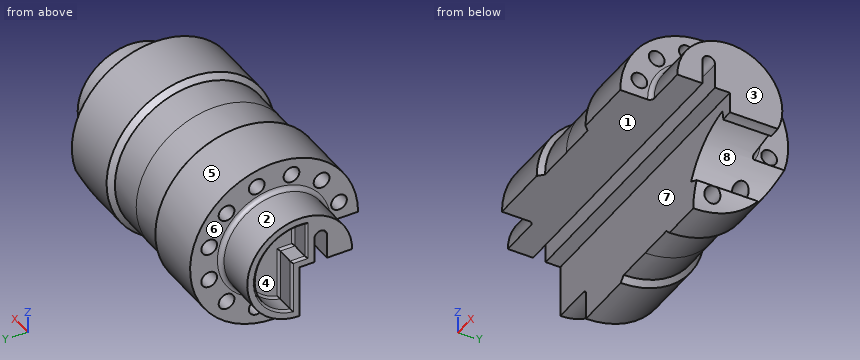
```python
from build123d import *

# Parameters (mm, degrees)
SKETCH2_W               = 86.249778207
SKETCH2_H               = 59.255694893
CUT_EXTRUDE1_DEPTH      = 1
CUT_EXTRUDE1_DEPTH_BACK = 139
CUT_EXTRUDE2_REACH      = 42
SKETCH4_R               = 3.75
CUT_EXTRUDE3_DEPTH      = 139
CUT_EXTRUDE4_DEPTH      = 10
FILLET1_R               = 1


with BuildPart() as part:
    # Sketch1 → Revolve1 (revolve)
    with BuildSketch(Plane(origin=(0, 0, 0), x_dir=(1, 0, 0), z_dir=(0, 1, 0))):
        with BuildLine():
            Line((-71.076656526, -28.85165756), (-71.076656526, -3.85165756))
            Line((-71.076656526, -3.85165756), (-52.076656526, -3.85165756))
            ThreePointArc((-52.076656526, -3.85165756), (-50.662442964, -3.265871122), (-50.076656526, -1.85165756))
            Line((-50.076656526, -1.85165756), (-50.076656526, 11.14834244))
            Line((-50.076656526, 11.14834244), (-21.576656526, 11.14834244))
            Line((-21.576656526, 11.14834244), (-19.076656526, 8.64834244))
            Line((-19.076656526, 8.64834244), (-1.576656526, 8.64834244))
            Line((-1.576656526, 8.64834244), (-1.576656526, -28.85165756))
            Line((-1.576656526, -28.85165756), (-71.076656526, -28.85165756))
        make_face()
    revolve1 = revolve(axis=Axis((-71.076656526, 0, 28.85165756), (1, 0, 0)))

    # Mirror6: Revolve1 across plane
    add(revolve1.mirror(Plane(origin=(-1.576656526, 0, 28.85165756), x_dir=(0, 0, 1), z_dir=(-1, 0, 0))))

    # Sketch2 → Cut-Extrude1 (cut, two sides)
    with BuildSketch(Plane.ZY.offset(71.076656526)) as cut_extrude1_sk:
        with Locations((-14.273231544, -29.627847447)):
            Rectangle(SKETCH2_W, SKETCH2_H)
        with BuildLine():
            Line((40.85165756, -13), (15.970307324, -13))
            ThreePointArc((15.970307324, -13), (12.970307324, -10), (15.970307324, -7))
            Line((15.970307324, -7), (40.85165756, -7))
            ThreePointArc((40.85165756, -7), (43.85165756, -10), (40.85165756, -13))
        make_face()
    extrude(amount=CUT_EXTRUDE1_DEPTH, mode=Mode.SUBTRACT)
    extrude(cut_extrude1_sk.sketch, amount=-CUT_EXTRUDE1_DEPTH_BACK, mode=Mode.SUBTRACT)

    # Sketch3 → Cut-Extrude2 (cut, up to next)
    with BuildSketch(Plane.XZ, mode=Mode.PRIVATE) as cut_extrude2_sk1:
        with BuildLine():
            ThreePointArc((61.845657255, 23.319928915), (46.616693458, 16.61902447), (36.202570927, 3.643296721))
            Line((36.202570927, 3.643296721), (40.734109863, 1.530205412))
            ThreePointArc((40.734109863, 1.530205412), (38.63446326, -4.655154022), (37.923343474, -11.14834244))
            Line((37.923343474, -11.14834244), (46.923343474, -11.14834244))
            Line((46.923343474, -11.14834244), (46.923343474, 1.85165756))
            ThreePointArc((46.923343474, 1.85165756), (47.509129911, 3.265871122), (48.923343474, 3.85165756))
            Line((48.923343474, 3.85165756), (67.923343474, 3.85165756))
            Line((67.923343474, 3.85165756), (67.923343474, 18.85165756))
            ThreePointArc((67.923343474, 18.85165756), (65.308671191, 18.737498502), (62.713898144, 18.39589015))
            Line((62.713898144, 18.39589015), (61.845657255, 23.319928915))
        make_face()
    cut_extrude2_tool1 = extrude(cut_extrude2_sk1.sketch, amount=-CUT_EXTRUDE2_REACH, mode=Mode.PRIVATE) & part.part
    add(cut_extrude2_tool1.solids().sort_by_distance((52.095068, 0, 8.03678))[0], mode=Mode.SUBTRACT)

    # Sketch4 → Cut-Extrude3 (cut)
    with BuildSketch(Plane.ZY.offset(71.076656526)):
        with Locations((20.569448116, 30.909626441)):
            Circle(SKETCH4_R)
        with Locations((37.133867003, 30.909626441)):
            Circle(SKETCH4_R)
        with Locations((51.479074558, 22.627416998)):
            Circle(SKETCH4_R)
        with Locations((59.761284001, 8.282209443)):
            Circle(SKETCH4_R)
        with Locations((59.761284001, -8.282209443)):
            Circle(SKETCH4_R)
        with Locations((51.479074558, -22.627416998)):
            Circle(SKETCH4_R)
        with Locations((37.133867003, -30.909626441)):
            Circle(SKETCH4_R)
        with Locations((20.569448116, -30.909626441)):
            Circle(SKETCH4_R)
        with Locations((6.224240562, -22.627416998)):
            Circle(SKETCH4_R)
        with Locations((-2.057968882, -8.282209443)):
            Circle(SKETCH4_R)
        with Locations((-2.057968882, 8.282209443)):
            Circle(SKETCH4_R)
        with Locations((6.224240562, 22.627416998)):
            Circle(SKETCH4_R)
    extrude(amount=-CUT_EXTRUDE3_DEPTH, mode=Mode.SUBTRACT)

    # Sketch6 → Cut-Extrude4 (cut)
    with BuildSketch(Plane.ZY.offset(71.076656526)):
        with BuildLine():
            Line((32.85165756, 4), (32.85165756, -3))
            Line((32.85165756, -3), (40.85165756, -3))
            Line((40.85165756, -3), (49.63626725, -3))
            ThreePointArc((49.63626725, -3), (32.352678431, 20.706106656), (8.236129431, 4))
            Line((8.236129431, 4), (32.85165756, 4))
        make_face()
    extrude(amount=-CUT_EXTRUDE4_DEPTH, mode=Mode.SUBTRACT)

    # Fillet1
    fillet1_edges = [part.edges().sort_by_distance(p)[0] for p in [
        (-61.076656526, -3, 41.243962405),
        (-61.076656526, 0.5, 32.85165756),
        (-61.076656526, 4, 20.543893496),
        (-61.076656526, 20.706106656, 32.352678431),
        (-71.076656526, -3, 41.243962405),
        (-71.076656526, 20.706106656, 32.352678431),
        (-71.076656526, 4, 20.543893496),
        (-71.076656526, 0.5, 32.85165756),
    ]]
    fillet(fillet1_edges, radius=FILLET1_R)


solid = part.part
```
Can you work these out from the model? Positions are in its coordinate system, mm. Face numbers are marked on the shaded views. A direction names the side the tool comes from. Give positions to 0.01 mm unless a question says otherwise; leave off trailing zeros. Order: outer loops, then holes, each group sorted by start corner. A loop starts at its lowest first (then second) coordinate and runs counter-clockwise, first axis right, second up. Notation, with made-up numbers: M 47,-17.75 L 68,-17.75 A36 cw 68,20.25 Z; hole C 87.25,-29 d10. An arc over 180 degrees is marked long. Write item = value, one per line. Start each with the question number.
Q1. Will these pins go through, and if not, where does the flat tip stop? pin 1 Ø10 at (y, z) = (30.91, 20.57) entering from -X; pin 2 Ø5 at (x, z) = (0, 12) entering from +Y; pin 3 Ø1.5 at (y, z) = (3.5, 57.5) entering from +X.
Q2. I need wall thicknesses on probe 1 along Y at (x, z) = (-22, 57); probe 2 along Z at (x, y) = (19, 5) (3 decimals); probe 3 along Z at (x, y) = (-26, 34). Which ranges of each line are inside material? Lowest first, please. Write a range as [from, to].
Q3. Suppose I cut it at B-B (x = 13.5). Count the separate pieces of the cut face and the enclosed holes in it, plus the area to 3 significant figures.
Q4. Suppose I cut it at A-A (x = -54). Write out the boundary of the cut face in (y, z), plus the area to 3 significant figures.
Q5. For the marked faces 5, 6, 7 and 8, which set-ups out of +Z, -Z, +X, -X, +Y, -Y let a thin tool reach every point of the face, with its end or its side?
Q6. We'd pull the mould along Z, two halves only. Please class the marked faces 1, 2, 3 and 4: pulls with the +Z half, pulls with the -Z half, needs draft (parallel to the pull), parting line crosses it, or undercut.
Check result:
q1.pin_1 = -50.08
q1.pin_2 = 34.65
q1.pin_3 = 46.92
q2.probe_1 = [-28.42, -10.82], [-5.74, 5.74], [10.82, 28.42]
q2.probe_2 = [-10.835, -3.872], [-0.244, 57.948], [61.575, 68.538]
q2.probe_3 = [7.78, 18.45], [22.69, 35.01], [39.26, 49.92]
q3.separate_pieces = 1
q3.enclosed_holes = 9
q3.area = 2,830 mm2
q4.outline = M -25,28.85 L -13,28.85 L -13,40.85 A3 cw -7,40.85 L -7,28.85 L 0,28.85 L 0,3.85 A25 ccw long Z
q4.area = 1,390 mm2
q5.face_5 = +X, -X
q5.face_6 = -X
q5.face_7 = -Z, +X, -X, -Y
q5.face_8 = +Y, -Y
q6.face_1 = pulls with the -Z half
q6.face_2 = parting line crosses it
q6.face_3 = needs draft
q6.face_4 = undercut
